Here's how the part is built. I have some questions about the finished solid (model axes, mm). A direction names the side the tool comes from. Round coordinates to 2 decimals unless told otherwise and drop trailing zeros. Write each loop counter-clockwise with the first axis right and the second up, starting at its lowest first coordinate (ties: lowest second). Pieces come first, ordered by that corner, then holes. Notation, with made-up numbers: (63.25, 62) - (109.25, 62) arc R17 ccw to (109.25, 70) - close; hole circle Ø3 at (-1.75, 35). An arc over 180 degrees is marked (long way). Write item = value, one per line. Start each with the question number.
Item 1: For P1, Ø1.5, axis at y = -10, z = 1, coming from the +X side; P2, Ø2, axis at y = -2, z = -1.5, coming from the +X side; P3, Ø2, axis at x = 3, y = -5.5, coming from the +Z side; P4, Ø1.4, axis at x = -9.48, z = 0, coming from the -Y side, each with a flat end and sliding along its axis, tell me the tip position at first contact or that it passes through.
Item 2: Thinking about a two-plate mould opening in X: for faces 3 (the face through (11.99, 0.99, -0.53)), 4 (the face through (-10.607, 1.014, -0.05)), 5 (the face through (3, 0, 0)), which applies, pulls with the +X half, pulls with the -X half, needs draft (parallel to the pull), parting line crosses it, or undercut?
Item 3: If we section it at D-D (x = 0): Please give me the cut outline in (y, z).
Item 4: Which directions (+Z, -Z, +X, -X, +Y, -Y) give clear straight access to the entire face, cutting with the end or side of a thin tool? Please do faces 1 (the face through (0, -12, 0)), 2 (the face through (-0.54, -5.92, 2.44)).
Item 5: If we section it at A-A (z = 0): Please give me the cut outline in (x, y), and give its area (3 significant figures).
Item 6: If we section it at B-B (x = -9.25): Please give me the cut outline in (y, z), and give its area (3 significant figures).
Item 7: If we section it at C-C (y = 1.25): Please give me the cut outline in (x, z), and give its area (3 significant figures).
Item 8: If I drill on line 1 along Y through (x, z) = (-9.5, 3.25); line 2 along X through (y, z) = (0.5, 6.5); line 3 along X through (y, z) = (-0.5, -1.25), over which ranges is the centre line in solid material (lowest first)? Write a range as [from, to].
Autodesk Inventor part; units mm, degrees
ref_plane "YZ Plane" through (0, 0, 0) normal (1, 0, 0) x (0, 1, 0)
ref_plane "XZ Plane" through (0, 0, 0) normal (0, 1, 0) x (-1, 0, 0)
ref_plane "XY Plane" through (0, 0, 0) normal (0, 0, 1) x (1, 0, 0)
sketch "Sketch1" plane through (0, 0, 0) normal (0, 1, 0) x (-1, 0, 0)
  circle A0 centre (0, 0) radius 12
  dimension "sa_diameter" = 24
extrude "Extrusion1" add sketch "Sketch1" along normal blind 2
sketch "Sketch2" plane through (0, 0, 0) normal (0, -1, 0) x (1, 0, 0)
  circle A0 centre (0, 0) radius 2.5
  dimension "d4" = 5
extrude "Extrusion2" add sketch "Sketch2" along normal blind 12
sketch "Sketch3" plane through (0, 2, 0) normal (0, 1, 0) x (1, 0, 0)
  circle A0 centre (-9.4812, 0) radius 1.1266
  point P0 (0, 0)
  dimension "d8" = 9.4812
  dimension "d9" = 2.2531
extrude "Extrusion3" cut sketch "Sketch3" against normal up to next
properties part number "Servo_arm"
Reply:
q1.P1 = 2.49
q1.P2 = 2.45
q1.P3 = 1.5
q1.P4 = through
q2.face_3 = parting line crosses it
q2.face_4 = undercut
q2.face_5 = needs draft
q3.outline = (-12, -2.5) - (0, -2.5) - (0, -12) - (2, -12) - (2, 12) - (0, 12) - (0, 2.5) - (-12, 2.5) - close
q4.face_1 = +Z, -Z, +X, -X, -Y
q4.face_2 = -Y
q5.outline = (-12, 0) - (-10.61, 0) - (-10.61, 2) - (-12, 2) - close; (-8.35, 0) - (-2.5, 0) - (-2.5, -12) - (2.5, -12) - (2.5, 0) - (12, 0) - (12, 2) - (-8.35, 2) - close
q5.area = 103 mm2
q6.outline = (0, -7.64) - (2, -7.64) - (2, -1.1) - (0, -1.1) - close; (0, 1.1) - (2, 1.1) - (2, 7.64) - (0, 7.64) - close
q6.area = 26.2 mm2
q7.outline = circle Ø24 at (0, 0); hole circle Ø2.25 at (-9.48, 0)
q7.area = 448 mm2
q8.line_1 = [0, 2]
q8.line_2 = [-10.09, 10.09]
q8.line_3 = [-2.17, 2.17]
